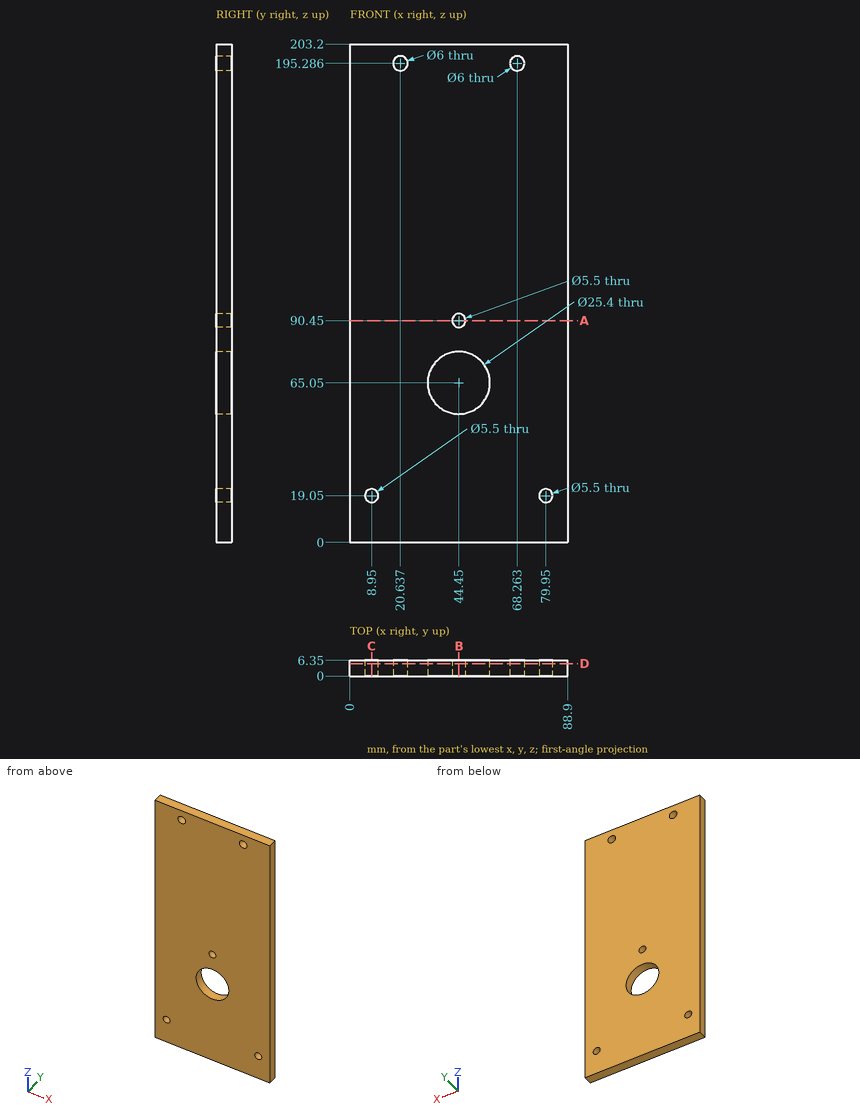
Source: three-view drawing plus pictorial views. Frame: mm from the lowest corner of the part. Give positions to 0.01 mm unless a question says otherwise; leave off trailing zeros. Order: outer loops, then holes, each group sorted by start corner. A loop starts at its lowest first (then second) coordinate and runs counter-clockwise, first axis right, second up. Notation, with made-up numbers: (-13, 86.25) -> (4, 86.25) arc R34 cw to (4, 124.25) -> close; hole circle Ø5 at (75, 56.25). An arc over 180 degrees is marked (long way). Write each question's results on one line, items separated by ' | '. Start each with the question number.
Item 1: Cut plane D-D on y = 5. Return the cut outline in (x, z), then the cut area to 3 significant figures.
Item 2: Cut plane B-B on x = 44.45. Return the cut outline in (y, z).
Item 3: Cut plane A-A on z = 90.45. Return the cut outline in (x, y).
Item 4: Line query: line 1 (Z direction, x = 44.45, y = 4.5); line 2 (X direction, y = 3.25, z = 19.05); line 3 (Z direction, x = 70.5, y = 1) (1 decimal). Output: solid intervals per line, ascending.
Item 5: Cut plane C-C on x = 8.95. Return the cut outline in (y, z).
Established:
1) outline: (0, 0) -> (88.9, 0) -> (88.9, 203.2) -> (0, 203.2) -> close; hole circle Ø5.5 at (8.95, 19.05); hole circle Ø6 at (20.64, 195.29); hole circle Ø25.4 at (44.45, 65.05); hole circle Ø5.5 at (44.45, 90.45); hole circle Ø6 at (68.26, 195.29); hole circle Ø5.5 at (79.95, 19.05) | area: 17,400 mm^2
2) outline: (0, 0) -> (6.35, 0) -> (6.35, 52.35) -> (0, 52.35) -> close; (0, 77.75) -> (6.35, 77.75) -> (6.35, 87.7) -> (0, 87.7) -> close; (0, 93.2) -> (6.35, 93.2) -> (6.35, 203.2) -> (0, 203.2) -> close
3) outline: (0, 0) -> (41.7, 0) -> (41.7, 6.35) -> (0, 6.35) -> close; (47.2, 0) -> (88.9, 0) -> (88.9, 6.35) -> (47.2, 6.35) -> close
4) line 1: 0 to 52.35, 77.75 to 87.7, 93.2 to 203.2 | line 2: 0 to 6.2, 11.7 to 77.2, 82.7 to 88.9 | line 3: 0 to 193.3, 197.3 to 203.2
5) outline: (0, 0) -> (6.35, 0) -> (6.35, 16.3) -> (0, 16.3) -> close; (0, 21.8) -> (6.35, 21.8) -> (6.35, 203.2) -> (0, 203.2) -> close
